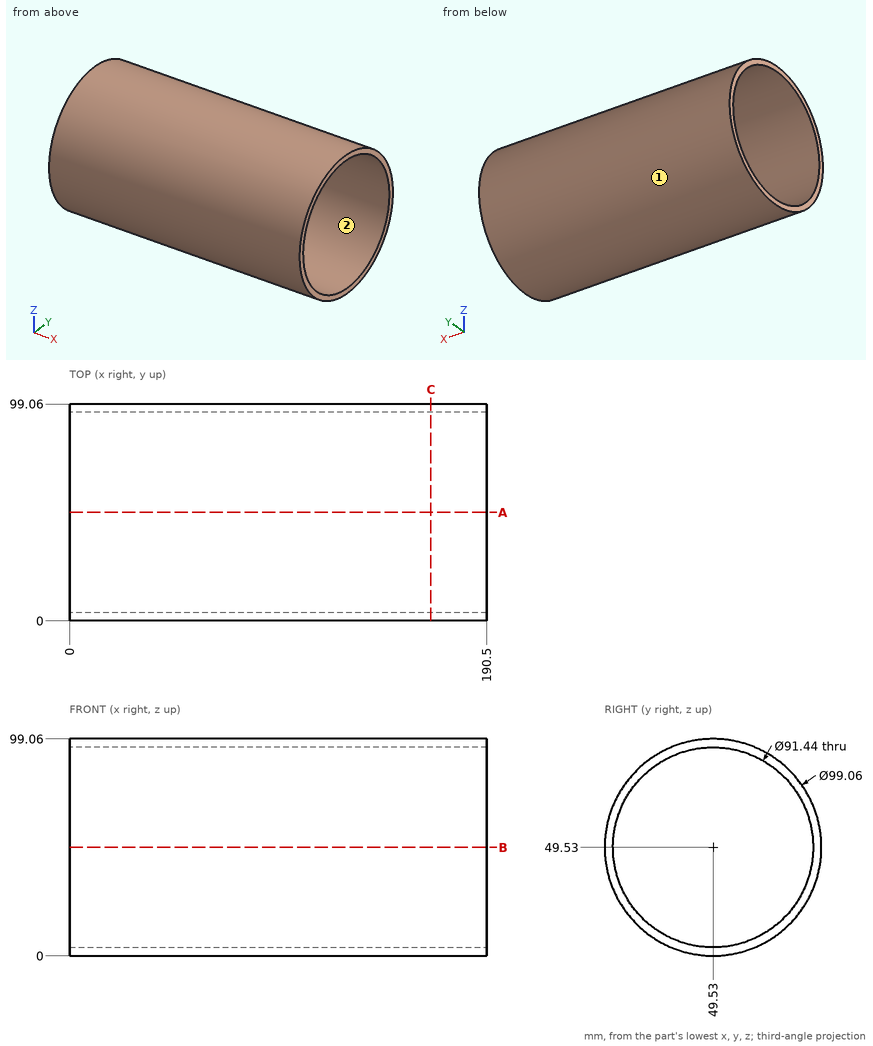
For this review, use the dimensioned drawing (mm, ordinates from the lowest corner) and the shaded views. Coordinates: 2 decimals unless noted, no trailing zeros. Write each loop counter-clockwise with the first axis right and the second up, starting at its lowest first coordinate (ties: lowest second). Pieces come first, ordered by that corner, then holes. Notation, with made-up numbers: (14, -0.75) -> (60, -0.75) arc R20 ccw to (60, 29.25) -> close; hole circle Ø4 at (28, -22.5). An arc over 180 degrees is marked (long way). Write each question's results on one line, items separated by ' | '. Start each with the question number.
(1) For line 1 along Y through (x, z) = (70, 49); line 2 along Z through (x, y) = (144, 59.5); line 3 along Y through (x, z) = (90, 40), list the stretches that pass through material, from the lowest coordinate up. Write a range as from..to.
(2) Take a section at A-A on y = 49.53. Write out the cut boundary in (x, z).
(3) Take a section at C-C on x = 165. Write out the cut boundary in (y, z), and give its area (3 significant figures).
(4) The part is to be moulded in two halves that separate along Z. For the marked faces 1 and 2, say which applies: pulls with the +Z half, pulls with the -Z half, needs draft (parallel to the pull), parting line crosses it, or undercut.
(5) Clearance check with flat-ended pins moving along their axes: P1, Ø2, axis at x = 151.5, y = 65, coming from the -Z side; P2, Ø12, axis at x = 161.5, y = 68, coming from the -Z side; P3, Ø4, axis at x = 100.5, z = 69, coming from the +Y side. State where each tip first meets the part, or that it passes through.
Results found:
1) line 1: y = 0..3.81, 95.25..99.06 | line 2: z = 1.01..4.91, 94.15..98.05 | line 3: y = 0.93..4.81, 94.25..98.13
2) outline: (0, 0) -> (190.5, 0) -> (190.5, 3.81) -> (0, 3.81) -> close; (0, 95.25) -> (190.5, 95.25) -> (190.5, 99.06) -> (0, 99.06) -> close
3) outline: circle Ø99.06 at (49.53, 49.53); hole circle Ø91.44 at (49.53, 49.53) | area: 1,140 mm2
4) face 1: parting line crosses it | face 2: undercut
5) P1: stops at z = 2.16 | P2: stops at z = 1.6 | P3: stops at y = 95.88
